Source: CAD feature listing. Evaluate the final solid. Frame: model axes, mm. A direction names the side the tool comes from. Round coordinates to 2 decimals unless told otherwise and drop trailing zeros. Write each loop counter-clockwise with the first axis right and the second up, starting at its lowest first coordinate (ties: lowest second). Pieces come first, ordered by that corner, then holes.
from build123d import *

# Parameters (mm, degrees)
BOSS_EXTRUDE1_DEPTH = 3
SKETCH2_R           = 1.5
CUT_EXTRUDE1_DEPTH  = 98.462813421
SKETCH3_W           = 15
SKETCH3_H           = 9
SKETCH3_W_2         = 3
SKETCH3_H_2         = 10
SKETCH3_H_3         = 3
CUT_EXTRUDE2_DEPTH  = 98.462813421


with BuildPart() as part:
    # Sketch1 → Boss-Extrude1 (new body)
    with BuildSketch(Plane(origin=(0, 0, 0), x_dir=(1, 0, 0), z_dir=(0, 1, 0))):
        with BuildLine():
            Line((-49, 79), (49, 79))
            ThreePointArc((49, 79), (54.656854249, 76.656854249), (57, 71))
            Line((57, 71), (57, -71))
            ThreePointArc((57, -71), (54.656854249, -76.656854249), (49, -79))
            Line((49, -79), (-49, -79))
            ThreePointArc((-49, -79), (-54.656854249, -76.656854249), (-57, -71))
            Line((-57, -71), (-57, 71))
            ThreePointArc((-57, 71), (-54.656854249, 76.656854249), (-49, 79))
        make_face()
    extrude(amount=BOSS_EXTRUDE1_DEPTH)

    # Sketch2 → Cut-Extrude1 (cut, through all)
    with BuildSketch(Plane(origin=(0, 3, 0), x_dir=(1, 0, 0), z_dir=(0, 1, 0))):
        with Locations(Location((-36.56, 3.04, 0), (0, 0, 270))):
            Circle(SKETCH2_R)
        with Locations(Location((-8.62, 3.04, 0), (0, 0, 270))):
            Circle(SKETCH2_R)
        with Locations(Location((-51.8, -47.76, 0), (0, 0, 270))):
            Circle(SKETCH2_R)
        with Locations(Location((-3.54, -49.03, 0), (0, 0, 270))):
            Circle(SKETCH2_R)
        with Locations(Location((34.95, 56.46, 0), (0, 0, 270))):
            Circle(SKETCH2_R)
        with Locations(Location((51.46, 56.46, 0), (0, 0, 270))):
            Circle(SKETCH2_R)
    extrude(amount=-CUT_EXTRUDE1_DEPTH, mode=Mode.SUBTRACT)

    # Sketch3 → Cut-Extrude2 (cut, through all)
    with BuildSketch(Plane(origin=(0, 0, 0), x_dir=(-1, 0, 0), z_dir=(0, -1, 0))):
        with Locations((27.5, -69.5)):
            Rectangle(SKETCH3_W, SKETCH3_H)
        with Locations((-27.5, -69.5)):
            Rectangle(SKETCH3_W, SKETCH3_H)
        with Locations((-2.5, -46.75)):
            Rectangle(SKETCH3_W_2, SKETCH3_H_2)
        with Locations((-2.5, -16.75)):
            Rectangle(SKETCH3_W_2, SKETCH3_H_2)
        with Locations((-27.5, 0)):
            Rectangle(SKETCH3_W, SKETCH3_H_3)
        with Locations((-52.5, -16.75)):
            Rectangle(SKETCH3_W_2, SKETCH3_H_2)
        with Locations((-52.5, -46.75)):
            Rectangle(SKETCH3_W_2, SKETCH3_H_2)
    extrude(amount=-CUT_EXTRUDE2_DEPTH, mode=Mode.SUBTRACT)


solid = part.part
1) Reachability of faces 1 (the face through (-54.719, 1.479, -76.594)), 2 (the face through (3, 1, 11.75)) from +Z, -Z, +X, -X, +Y, -Y: full face, straight path, thin tool, end or side. Return the list, or none.
Taken from the geometry:
face 1: -Z, -X, +Y, -Y
face 2: +Y, -Y
2) Pull-direction query (Z, two-part tool) for faces 3 (the face through (35, 1, 70)), 4 (the face through (-54.594, 1.479, 76.719)), 5 (the face through (1, 0, -1)); classes: released by +Z, released by -Z, zero draft, split by the parting line, or undercut.
Taken from the geometry:
face 3: undercut
face 4: released by +Z
face 5: zero draft
3) Material intervals for line 1 (X direction, y = 1.55, z = -3.04); line 2 (X direction, y = 2.25, z = -56.46); line 3 (Z direction, x = 1.5, y = 2.4), sorted ascending.
Taken from the geometry:
line 1: x = -57 to -38.06, -35.06 to -10.12, -7.12 to 57
line 2: x = -57 to 33.45, 36.45 to 49.96, 52.96 to 57
line 3: z = -79 to 11.75, 21.75 to 41.75, 51.75 to 79
4) Contact query for a flat-ended pin moving along its axis: P1, Ø2.5, axis at x = -3.54, z = 49.03, coming from the -Y side (3 decimals). Output: stop coordinate, or through.
Taken from the geometry:
P1: passes through
5) Section query A-A on x = -33. Return the cut outline in (y, z).
Taken from the geometry:
outline: (0, -79) - (3, -79) - (3, 65) - (0, 65) - close; (0, 74) - (3, 74) - (3, 79) - (0, 79) - close
6) Section query B-B on y = 1. State how many separate pieces and enclosed holes the cut face has, then the cut area to 3 significant figures.
Taken from the geometry:
separate pieces: 1
enclosed holes: 13
area: 17,500 mm2
